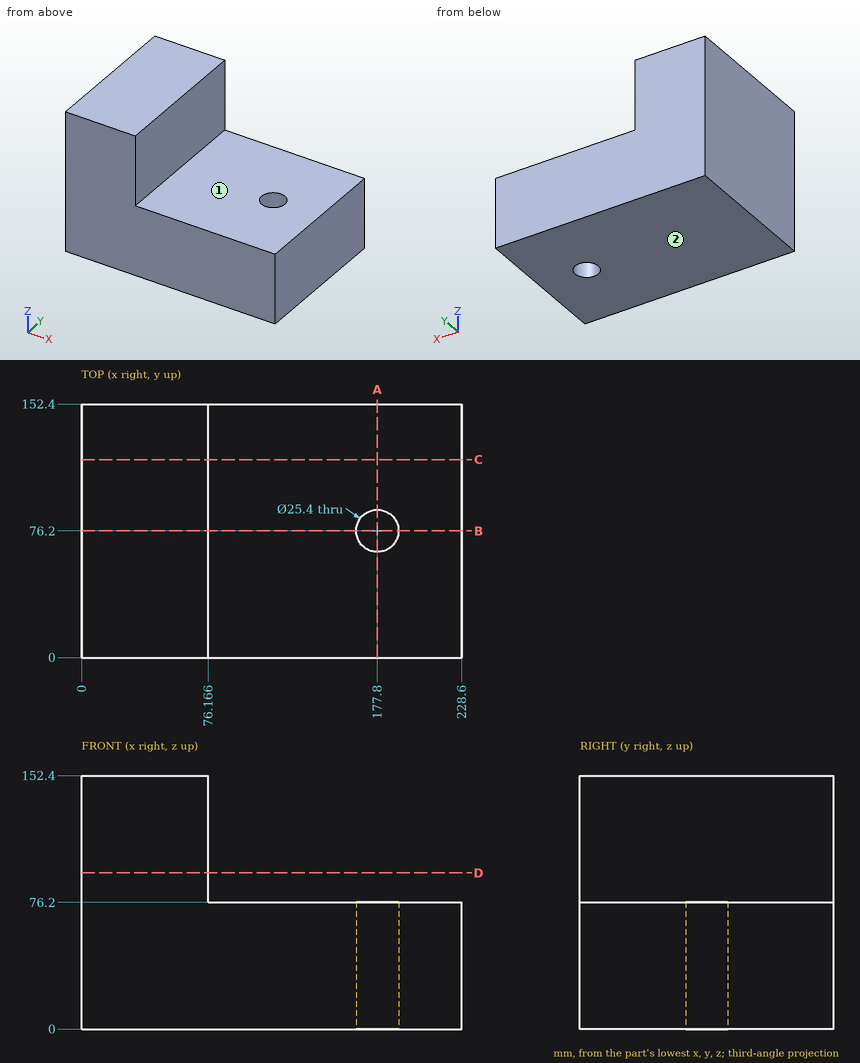
Check sheet for the drawn part. Datum: minimum x, y, z corner. Units: mm. A direction names the side the tool comes from. Coordinates: 2 decimals unless noted, no trailing zeros. Order: outer loops, then holes, each group sorted by start corner. A loop starts at its lowest first (then second) coordinate and runs counter-clockwise, first axis right, second up. Notation, with made-up numbers: (-26.5, 67) -> (22.5, 67) arc R21 cw to (22.5, 91) -> close; hole circle Ø3 at (9.25, 27.5). An arc over 180 degrees is marked (long way). Use a Markdown table: item, result. Add a question column.
1. Cross-section at A-A (x = 177.8). Enter the section's corners in (y, z).
2. Set-up check for the marked faces 1 and 2: record each of +Z, -Z, +X, -X, +Y, -Y from which the full face is reachable in a straight line by a thin tool's end or side.
3. Material ranges on L1, parallel to Y at x = 177.8, z = 55; L2, parallel to Z at x = 86, y = 85; L3, parallel to X at y = 76, z = 41, recorded low to high.
4. Cross-section at D-D (z = 94). Enter the section's corners in (x, y).
5. Go/stop test with flat-tipped pins: pin 1 Ø6 at (y, z) = (45.5, 122.5) entering from -X; pin 2 Ø1 at (y, z) = (47, 106.5) entering from +X; pin 3 Ø5 at (x, y) = (103, 73.5) entering from +Z. Record where each tip stops, or that it passes through.
6. Cross-section at C-C (y = 119). Enter the section's corners in (x, z), and give its area (3 significant figures).
7. Cross-section at B-B (y = 76.2). Enter the section's corners in (x, z), and give its area (3 significant figures).
Filled sheet:
| question | item | result |
|---|---|---|
| 1 | outline | (0, 0) -> (63.5, 0) -> (63.5, 76.2) -> (0, 76.2) -> close; (88.9, 0) -> (152.4, 0) -> (152.4, 76.2) -> (88.9, 76.2) -> close |
| 2 | face 1 | +Z, +X, +Y, -Y |
| 2 | face 2 | -Z, +X, -X, +Y, -Y |
| 3 | L1 | 0 to 63.5, 88.9 to 152.4 |
| 3 | L2 | 0 to 76.2 |
| 3 | L3 | 0 to 165.1, 190.5 to 228.6 |
| 4 | outline | (0, 0) -> (76.17, 0) -> (76.17, 152.4) -> (0, 152.4) -> close |
| 5 | pin 1 | x = 0 |
| 5 | pin 2 | x = 76.17 |
| 5 | pin 3 | z = 76.2 |
| 6 | outline | (0, 0) -> (228.6, 0) -> (228.6, 76.2) -> (76.17, 76.2) -> (76.17, 152.4) -> (0, 152.4) -> close |
| 6 | area | 23,200 mm2 |
| 7 | outline | (0, 0) -> (165.1, 0) -> (165.1, 76.2) -> (76.17, 76.2) -> (76.17, 152.4) -> (0, 152.4) -> close; (190.5, 0) -> (228.6, 0) -> (228.6, 76.2) -> (190.5, 76.2) -> close |
| 7 | area | 21,300 mm2 |
